Autodesk Inventor part; units mm, degrees
ref_plane "YZ Plane" through (0, 0, 0) normal (1, 0, 0) x (0, 1, 0)
ref_plane "XZ Plane" through (0, 0, 0) normal (0, 1, 0) x (-1, 0, 0)
ref_plane "XY Plane" through (0, 0, 0) normal (0, 0, 1) x (1, 0, 0)
sketch "Эскиз1" plane through (0, 0, 0) normal (0, 0, 1) x (1, 0, 0)
  point P0 (0, 0)
sketch "Эскиз2" plane through (0, 0, 0) normal (0, 1, 0) x (-1, 0, 0)
  line L0 (0, 18.4752) -> (16, 9.2376)
  line L1 (16, 9.2376) -> (16, -9.2376)
  line L2 (16, -9.2376) -> (0, -18.4752)
  line L3 (0, -18.4752) -> (-16, -9.2376)
  line L4 (-16, -9.2376) -> (-16, 9.2376)
  line L5 (-16, 9.2376) -> (0, 18.4752)
  circle A0 centre (0, 0) radius 5.5
  dimension "d0" = 32
  dimension "d1" = 11
extrude "Выдавливание1" add sketch "Эскиз2" along normal blind 5.5
sketch "Эскиз3" plane through (0, 5.5, 0) normal (0, 1, 0) x (1, 0, 0)
  circle A0 centre (0, 0) radius 5.5
  circle A1 centre (0, 0) radius 10
  dimension "d4" = 20
extrude "Выдавливание2" add sketch "Эскиз3" along normal blind 2.5
chamfer "Фаска1" distance 1 angle 45 1 edges at (-10, 8, 0) measured on face at (8.3499, 8, 1.2365)
sketch "Эскиз4" plane through (0, 0, 0) normal (0, -1, 0) x (1, 0, 0)
  circle A0 centre (0, 0) radius 5.5
  circle A1 centre (0, 0) radius 11.75
  dimension "d10" = 23.5
extrude "Выдавливание3" add sketch "Эскиз4" along normal blind 3
sketch "Эскиз5" plane through (0, -3, 0) normal (0, -1, 0) x (1, 0, 0)
  circle A0 centre (0, 0) radius 11.75
  circle A1 centre (0, 0) radius 13.5
  dimension "d13" = 27
extrude "Выдавливание4" add sketch "Эскиз5" along normal blind 8
sketch "Эскиз6" plane through (0, -3, 0) normal (0, -1, 0) x (1, 0, 0)
  circle A0 centre (0, 0) radius 5.5
  circle A1 centre (0, 0) radius 11.75
extrude "Выдавливание5" add sketch "Эскиз6" along normal blind 8
thread "Резьба1"
chamfer "Фаска2" distance 2 angle 45 1 edges at (-13.5, -11, 0) measured on face at (12.6721, -11, -2.0142)
chamfer "Фаска3" distance 1.75 angle 45 1 edges at (-13.5, -3, 0)
fillet "Сопряжение1" radius 0.5 2 edges at (-11.7501, -3, 0) (-11.75, -3, 0)
fillet "Сопряжение2" radius 1 1 edges at (-11.75, 0, 0)
Can you work these out from the model? Positions are in its coordinate system, mm. A direction names the side the tool comes from. Coordinates: 2 decimals unless noted, no trailing zeros. Loops run counter-clockwise (first coordinate to the right, second up) from the corner with the lowest first, then second, coordinate; pieces in that order, holes last. Notation, with made-up numbers: (-15, 61) - (20, 61) arc R15 cw to (20, 82) - close; hole circle Ø3 at (81.25, 1.5). An arc over 180 degrees is marked (long way). Answer as CSV lines item,"result". Start each with the question number.
1) Which directions (+Z, -Z, +X, -X, +Y, -Y) give clear straight access to the entire face, cutting with the end or side of a thin tool? Please do faces 1 (the cylindrical face through (-2.93, -6.85, 13.18)), 2 (the flat face through (-7, 5.5, -8)), 3 (the flat face through (-8.1, 2.7, -13.8)).
2) Thinking about a two-plate mould opening in Y: for faces 4 (the flat face through (-4, 8, 4)), 5 (the cylindrical face through (11.207, -1.884, -3.529)), 6 (the flat face through (5, -11, -3)), 7 (the flat face through (7.89, 2.71, -13.92)), which applies, pulls with the +Y half, pulls with the -Y half, needs draft (parallel to the pull), parting line crosses it, or undercut?
3) For pin 1 (6.5 mm diameter, centred on x = 0, z = 0, fed in from +Y); pin 2 (5 mm diameter, centred on y = -6.5, z = 9, fed in from +X); pin 3 (1.5 mm diameter, centred on x = 0.5, y = -7, fed in from +Z); pin 4 (10 mm diameter, centred on x = 6.5, y = -9, fed in from -Z), each with a flat end and sliding along its axis, tell me the tip position at first contact or that it passes through.
4) Suppose I cut it at A-A (y = -0.5). Please give me the cut outline in (x, z), plus the area to 3 significant figures.
5) Suppose I cut it at B-B (z = -16). Please give me the cut outline in (x, y).
6) I need wall thicknesses on line 1 (Z direction, x = 0, y = -2.25); line 2 (Y direction, x = -11, z = -6.5); line 3 (Z direction, x = 4.5, y = -2.5). Which ranges of each line are inside material? Lowest first, please. Write a range as from..to.
Check result:
1,face 1,"-Y"
1,face 2,"+Y"
1,face 3,"-Z, -X, +Y, -Y"
2,face 4,"pulls with the +Y half"
2,face 5,"undercut"
2,face 6,"pulls with the -Y half"
2,face 7,"needs draft"
3,pin 1,"passes through"
3,pin 2,"stops at x = 11.83"
3,pin 3,"stops at z = 13.5"
3,pin 4,"stops at z = -13.42"
4,outline,"circle Ø23.77 at (0, 0); hole circle Ø11 at (0, 0)"
4,area,"349 mm²"
5,outline,"(-4.29, 0) - (4.29, 0) - (4.29, 5.5) - (-4.29, 5.5) - close"
6,line 1,"z = -11.75..-5.5, 5.5..11.75"
6,line 2,"y = -9.72..-4.03, 0..5.5"
6,line 3,"z = -10.85..-3.16, 3.16..10.85"
